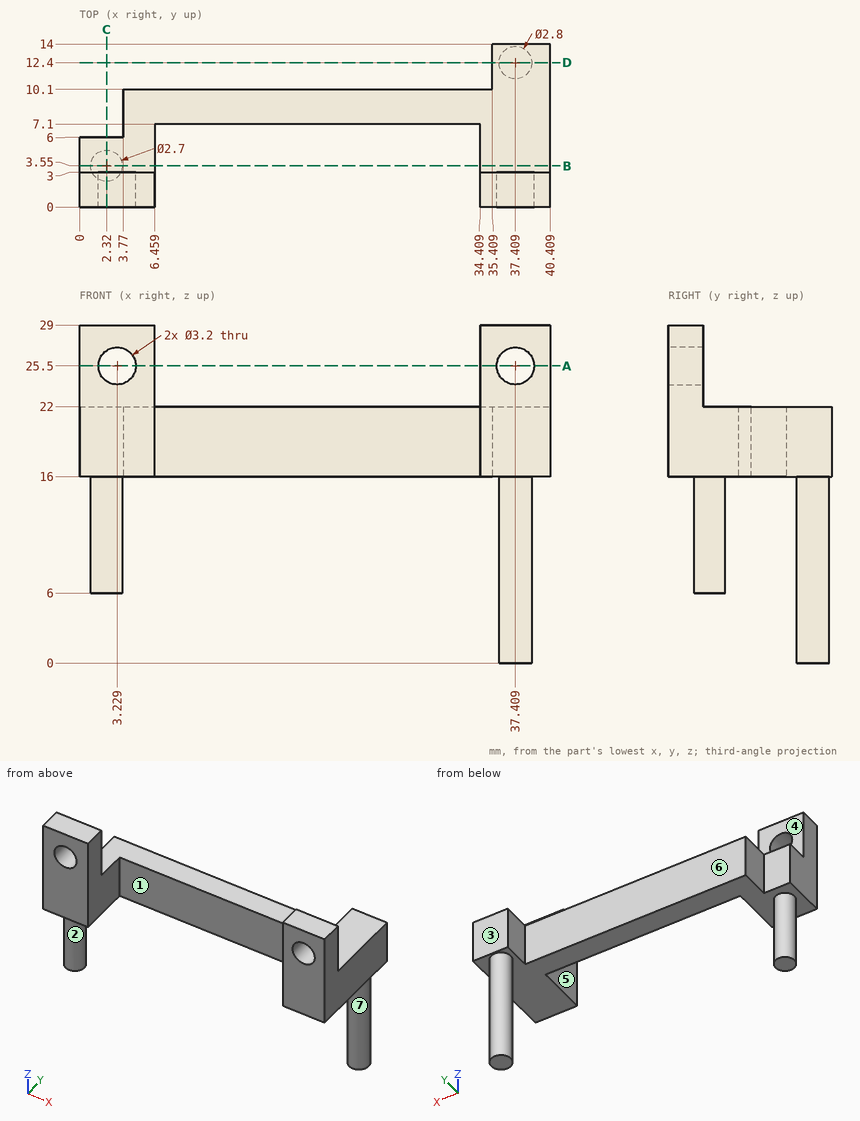
The drawing under review shows one solid part. Ordinate dimensions are in mm from its lowest x, y, z. A direction names the side the tool comes from. Coordinates: 2 decimals unless noted, no trailing zeros. Order: outer loops, then holes, each group sorted by start corner. A loop starts at its lowest first (then second) coordinate and runs counter-clockwise, first axis right, second up. Notation, with made-up numbers: (19.5, 5.25) -> (54.5, 5.25) arc R19 ccw to (54.5, 34.25) -> close; hole circle Ø2 at (89, 7.5). An arc over 180 degrees is marked (long way). Answer as CSV lines item,"result".
Q1. We need section A-A (z = 25.5). State the section outline as (x, y) points.
Model answer:
outline,"(0, 0) -> (1.63, 0) -> (1.63, 3) -> (0, 3) -> close; (4.83, 0) -> (6.46, 0) -> (6.46, 3) -> (4.83, 3) -> close; (34.41, 0) -> (35.81, 0) -> (35.81, 3) -> (34.41, 3) -> close; (39.01, 0) -> (40.41, 0) -> (40.41, 3) -> (39.01, 3) -> close"
Q2. Clearance check with flat-ended pins moving along their axes: pin 1 Ø7 at (x, y) = (23, 4.5) entering from -Z; pin 2 Ø3 at (x, z) = (39, 25.5) entering from +Y; pin 3 Ø2 at (y, z) = (4, 9) entering from +X; pin 4 Ø1.5 at (x, y) = (11, 11) entering from -Z. State where each tip first meets the part, or that it passes through.
Model answer:
pin 1,"stops at z = 16"
pin 2,"stops at y = 3"
pin 3,"stops at x = 3.67"
pin 4,"passes through"
Q3. For the marked faces 4, 5, 6 and 7, list the 3-axis set-ups (+Z, -Z, +X, -X, +Y, -Y) from which the entire face can be reached by the end or side of a thin tool; tool diameter is ignored.
Model answer:
face 4,"+Z, +X, -X, +Y"
face 5,"+Z, -Z, -Y"
face 6,"+Z, -Z, -X, +Y"
face 7,"-Z"
Q4. Wall thickness on line 1 along X through (y, z) = (1.3, 25.5); line 2 along X through (y, z) = (1.5, 20.25); line 3 along Z through (x, y) = (2, 4.5): over which ranges is each line inside the solid? List them lowest first. Write a range as [from, to].
Model answer:
line 1,"x = [0, 1.63], [4.83, 6.46], [34.41, 35.81], [39.01, 40.41]"
line 2,"x = [0, 6.46], [34.41, 40.41]"
line 3,"z = [6, 22]"
Q5. We need section C-C (x = 2.32). State the section outline as (y, z) points.
Model answer:
outline,"(0, 16) -> (2.2, 16) -> (2.2, 6) -> (4.9, 6) -> (4.9, 16) -> (6, 16) -> (6, 22) -> (3, 22) -> (3, 24.18) -> (0, 24.18) -> close; (0, 26.82) -> (3, 26.82) -> (3, 29) -> (0, 29) -> close"
Q6. We need section B-B (y = 3.55). State the section outline as (x, z) points.
Model answer:
outline,"(0, 16) -> (0.97, 16) -> (0.97, 6) -> (3.67, 6) -> (3.67, 16) -> (6.46, 16) -> (6.46, 22) -> (0, 22) -> close; (34.41, 16) -> (40.41, 16) -> (40.41, 22) -> (34.41, 22) -> close"
Q7. Draft analysis for pull direction X (two halves, no side actions). For the marked faces 1, 2 and 3, state which applies: released by +X, released by -X, zero draft, split by the parting line, or undercut.
Model answer:
face 1,"undercut"
face 2,"split by the parting line"
face 3,"zero draft"
Q8. We need section D-D (y = 12.4). State the section outline as (x, z) points.
Model answer:
outline,"(35.41, 16) -> (36.01, 16) -> (36.01, 0) -> (38.81, 0) -> (38.81, 16) -> (40.41, 16) -> (40.41, 22) -> (35.41, 22) -> close"
